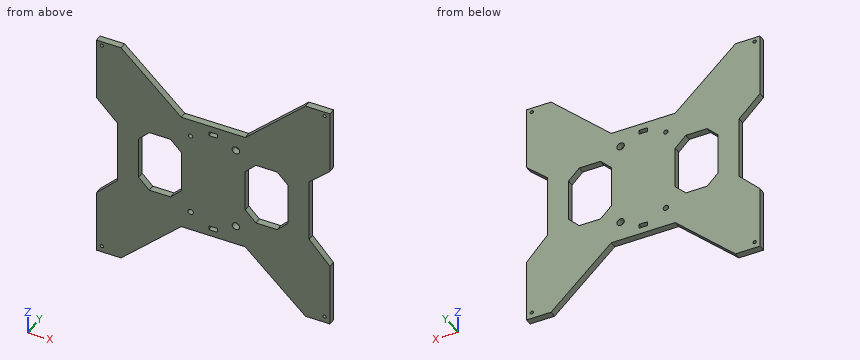
from build123d import *

# Parameters (mm, degrees)
BOSS_EXTRUDE1_DEPTH = 6.3
SKETCH3_W           = 8
SKETCH3_H           = 4
SKETCH3_W_2         = 40
SKETCH3_H_2         = 60
CUT_EXTRUDE1_DEPTH  = 310.776839031
CHAMFER1_SIZE       = 10
SKETCH4_R           = 1.55
SKETCH4_R_2         = 2.55
SKETCH4_R_3         = 2.05
SKETCH4_R_4         = 3.5
CUT_EXTRUDE2_DEPTH  = 310.776839031


with BuildPart() as part:
    # Sketch1 → Boss-Extrude1 (new body)
    with BuildSketch(Plane(origin=(0, 0, 0), x_dir=(1, 0, 0), z_dir=(0, 1, 0))):
        Polygon((0, 0), (23, 0), (79.5, 52.5), (139.5, 52.5), (196, 0), (219, 0), (219, 60), (199.5, 77.642351694), (199.5, 137.642351694), (219, 159), (219, 219), (196, 219), (139.5, 166.5), (79.5, 166.5), (23, 219), (0, 219), (0, 159), (19.5, 139.5), (19.5, 79.5), (0, 60), align=None)
    extrude(amount=BOSS_EXTRUDE1_DEPTH)

    # Sketch3 → Cut-Extrude1 (cut, through all)
    with BuildSketch(Plane(origin=(0, 6.3, 0), x_dir=(1, 0, 0), z_dir=(0, 1, 0))):
        with Locations((109.5, 158.5)):
            Rectangle(SKETCH3_W, SKETCH3_H)
        with Locations((109.5, 60.5)):
            Rectangle(SKETCH3_W, SKETCH3_H)
        with Locations((59.5, 109.087189265)):
            Rectangle(SKETCH3_W_2, SKETCH3_H_2)
        with Locations((159.5, 108.055162429)):
            Rectangle(SKETCH3_W_2, SKETCH3_H_2)
    extrude(amount=-CUT_EXTRUDE1_DEPTH, mode=Mode.SUBTRACT)

    # Chamfer1
    chamfer1_edges = [part.edges().sort_by_distance(p)[0] for p in [
        (79.5, 3.15, -139.087189265),
        (79.5, 3.15, -79.087189265),
        (39.5, 3.15, -79.087189265),
        (39.5, 3.15, -139.087189265),
        (179.5, 3.15, -138.055162429),
        (179.5, 3.15, -78.055162429),
        (139.5, 3.15, -78.055162429),
        (139.5, 3.15, -138.055162429),
    ]]
    chamfer(chamfer1_edges, length=CHAMFER1_SIZE)

    # Sketch4 → Cut-Extrude2 (cut, through all)
    with BuildSketch(Plane(origin=(0, 6.3, 0), x_dir=(1, 0, 0), z_dir=(0, 1, 0))):
        with Locations(Location((5, 213.071175847, 0), (0, 0, 270))):
            Circle(SKETCH4_R)
        with Locations(Location((214, 213.071175847, 0), (0, 0, 270))):
            Circle(SKETCH4_R)
        with Locations(Location((214, 4.071175847, 0), (0, 0, 270))):
            Circle(SKETCH4_R)
        with Locations(Location((5, 4.071175847, 0), (0, 0, 270))):
            Circle(SKETCH4_R)
        with Locations(Location((88.25, 148.071175847, 0), (0, 0, 270))):
            Circle(SKETCH4_R_2)
        with Locations(Location((88.25, 69.071175847, 0), (0, 0, 270))):
            Circle(SKETCH4_R_3)
        with Locations(Location((130.75, 69.071175847, 0), (0, 0, 270))):
            Circle(SKETCH4_R_4)
        with Locations(Location((130.75, 148.071175847, 0), (0, 0, 270))):
            Circle(SKETCH4_R_4)
    extrude(amount=-CUT_EXTRUDE2_DEPTH, mode=Mode.SUBTRACT)


solid = part.part
For this review, take the finished solid that the model builds, in its own axes (mm). Round coordinates to 2 decimals unless told otherwise and drop trailing zeros. Write each loop counter-clockwise with the first axis right and the second up, starting at its lowest first coordinate (ties: lowest second). Pieces come first, ordered by that corner, then holes. Notation, with made-up numbers: (15, -33) - (55, -33) arc R22 ccw to (55, 2) - close; hole circle Ø6 at (51.5, -10.75). An arc over 180 degrees is marked (long way). Use a Markdown table: item, result.
Q1. We need section B-B (z = -38.5). Give the boundary of the cut face in (x, y), plus the area to 3 significant figures.
Derived:
| item | result |
|---|---|
| outline | (0, 0) - (64.43, 0) - (64.43, 6.3) - (0, 6.3) - close; (154.57, 0) - (219, 0) - (219, 6.3) - (154.57, 6.3) - close |
| area | 812 mm2 |
Q2. Wall thickness on line 1 along X through (y, z) = (6.25, -116); line 2 along Z through (x, y) = (130.75, 3.5); line 3 along X through (y, z) = (5, -85.5): over which ranges is each line inside the solid? List them lowest first.
Derived:
| item | result |
|---|---|
| line 1 | x = 19.5 to 39.5, 79.5 to 139.5, 179.5 to 199.5 |
| line 2 | z = -166.5 to -151.57, -144.57 to -72.57, -65.57 to -52.5 |
| line 3 | x = 19.5 to 43.09, 75.91 to 142.06, 176.94 to 199.5 |
Q3. Clearance check with flat-ended pins moving along their axes: pin 1 (6.5 mm diameter, centred on x = 88.25, z = -69.07, fed in from +Y); pin 2 (3 mm diameter, centred on y = 3.5, z = -120.5, fed in from +X); pin 3 (3 mm diameter, centred on x = 141, y = 4, fed in from +Z); pin 4 (2 mm diameter, centred on x = 177.5, y = 1, fed in from +Z). State where each tip first meets the part, or that it passes through.
Derived:
| item | result |
|---|---|
| pin 1 | stops at y = 6.3 |
| pin 2 | stops at x = 199.5 |
| pin 3 | stops at z = -49.71 |
| pin 4 | stops at z = -16.26 |
Q4. We need section D-D (z = -135). Give the boundary of the cut face in (x, y), plus the area to 3 significant figures.
Derived:
| item | result |
|---|---|
| outline | (19.5, 0) - (45.41, 0) - (45.41, 6.3) - (19.5, 6.3) - close; (73.59, 0) - (146.44, 0) - (146.44, 6.3) - (73.59, 6.3) - close; (172.56, 0) - (199.5, 0) - (199.5, 6.3) - (172.56, 6.3) - close |
| area | 792 mm2 |
Q5. We need section C-C (x = 75.5). Give the boundary of the cut face in (y, z), plus the area to 3 significant figures.
Derived:
| item | result |
|---|---|
| outline | (0, -170.22) - (6.3, -170.22) - (6.3, -133.09) - (0, -133.09) - close; (0, -85.09) - (6.3, -85.09) - (6.3, -48.78) - (0, -48.78) - close |
| area | 463 mm2 |
Q6. We need section A-A (x = 130.75). Give the boundary of the cut face in (y, z).
Derived:
| item | result |
|---|---|
| outline | (0, -166.5) - (6.3, -166.5) - (6.3, -151.57) - (0, -151.57) - close; (0, -144.57) - (6.3, -144.57) - (6.3, -72.57) - (0, -72.57) - close; (0, -65.57) - (6.3, -65.57) - (6.3, -52.5) - (0, -52.5) - close |
